Geometry: final body of the model. Coordinates: model frame, mm. A direction names the side the tool comes from. Give positions to 0.01 mm unless a question says otherwise; leave off trailing zeros. Loops run counter-clockwise (first coordinate to the right, second up) from the corner with the lowest first, then second, coordinate; pieces in that order, holes last. Notation, with made-up numbers: (24.5, -34) -> (66.5, -34) arc R17 ccw to (66.5, -7) -> close; hole circle Ø10 at (62.25, 48). An arc over 180 degrees is marked (long way). Answer in a Markdown table with one row per item. Add a question column.
1) Draft query along Z for faces 3 (the flat face through (75, 3, 0)), 4 (the flat face through (75, 5.08, -19)), 5 (the flat face through (116, 3, -12.7)). Return one class per face: +Z half, -Z half, draft (parallel to the pull), parting line (faces both ways), or undercut.
2) Section query D-D (x = 16). Return the cut outline in (y, z), plus the area to 3 significant figures.
3) Line query: line 1 (Z direction, x = 19.5, y = 4.1); line 2 (X direction, y = 4.85, z = -25); line 3 (X direction, y = 4.55, z = -21). Output: solid intervals per line, ascending. Write a range as from..to.
4) Section query C-C (z = -14.5). Return the cut outline in (x, y).
5) First-contact query: P1, Ø1.5, axis at x = 117.5, y = 4, coming from the +Z side. Flat tip, straight axial feed; report the tip coordinate or a pass-through.
6) Access query for faces 1 (the flat face through (21, 3, -12.7)), 2 (the flat face through (75, 0, -19)). Directions: +Z, -Z, +X, -X, +Y, -Y. A direction counts if a zero-diameter tool reaches every point of the face in a straight line with its end or side. Return the directions, or none.
7) Section query A-A (y = 3.25). Return the cut outline in (x, z), plus the area to 3 significant figures.
8) Section query B-B (x = 117). Return the cut outline in (y, z), plus the area to 3 significant figures.
```python
from build123d import *

# Parameters (mm, degrees)
SKETCH1_W           = 152.4
SKETCH1_H           = 38.1
BOSS_EXTRUDE1_DEPTH = 5.08
CUT_EXTRUDE1_DEPTH  = 158.172441605
CUT_EXTRUDE3_DEPTH  = 158.172441605


with BuildPart() as part:
    # Sketch1 → Boss-Extrude1 (new body)
    with BuildSketch(Plane(origin=(0, 0, 0), x_dir=(1, 0, 0), z_dir=(0, 1, 0))):
        with Locations((76.2, 19.05)):
            Rectangle(SKETCH1_W, SKETCH1_H)
    extrude(amount=BOSS_EXTRUDE1_DEPTH)

    # Sketch2 → Cut-Extrude1 (cut, through all)
    with BuildSketch(Plane(origin=(0, 5.08, 0), x_dir=(1, 0, 0), z_dir=(0, 1, 0))):
        Polygon((25.049816881, 12.7), (28.71599109, 19.05), (25.049816881, 25.4), (17.717468462, 25.4), (14.051294253, 19.05), (17.717468462, 12.7), align=None)
    extrude(amount=-CUT_EXTRUDE1_DEPTH, mode=Mode.SUBTRACT)

    # Sketch5 → Cut-Extrude3 (cut, through all)
    with BuildSketch(Plane(origin=(0, 5.08, 0), x_dir=(1, 0, 0), z_dir=(0, 1, 0))):
        Polygon((119.853560994, 25.4), (112.521212575, 25.4), (108.855038366, 19.05), (112.521212575, 12.7), (119.853560994, 12.7), (123.519735203, 19.05), align=None)
    extrude(amount=-CUT_EXTRUDE3_DEPTH, mode=Mode.SUBTRACT)


solid = part.part
```
Evaluation:
| question | item | result |
|---|---|---|
| 1 | face 3 | +Z half |
| 1 | face 4 | draft |
| 1 | face 5 | undercut |
| 2 | outline | (0, -38.1) -> (5.08, -38.1) -> (5.08, -22.43) -> (0, -22.43) -> close; (0, -15.67) -> (5.08, -15.67) -> (5.08, 0) -> (0, 0) -> close |
| 2 | area | 159 mm² |
| 3 | line 1 | -38.1..-25.4, -12.7..0 |
| 3 | line 2 | 0..17.49, 25.28..112.29, 120.08..152.4 |
| 3 | line 3 | 0..15.18, 27.59..109.98, 122.39..152.4 |
| 4 | outline | (0, 0) -> (16.68, 0) -> (16.68, 5.08) -> (0, 5.08) -> close; (26.09, 0) -> (111.48, 0) -> (111.48, 5.08) -> (26.09, 5.08) -> close; (120.89, 0) -> (152.4, 0) -> (152.4, 5.08) -> (120.89, 5.08) -> close |
| 5 | P1 | z = 0 |
| 6 | face 1 | +Y, -Y |
| 6 | face 2 | +Z, -Z, +X, -X, -Y |
| 7 | outline | (0, -38.1) -> (152.4, -38.1) -> (152.4, 0) -> (0, 0) -> close; hole (14.05, -19.05) -> (17.72, -25.4) -> (25.05, -25.4) -> (28.72, -19.05) -> (25.05, -12.7) -> (17.72, -12.7) -> close; hole (108.86, -19.05) -> (112.52, -25.4) -> (119.85, -25.4) -> (123.52, -19.05) -> (119.85, -12.7) -> (112.52, -12.7) -> close |
| 7 | area | 5,530 mm² |
| 8 | outline | (0, -38.1) -> (5.08, -38.1) -> (5.08, -25.4) -> (0, -25.4) -> close; (0, -12.7) -> (5.08, -12.7) -> (5.08, 0) -> (0, 0) -> close |
| 8 | area | 129 mm² |
